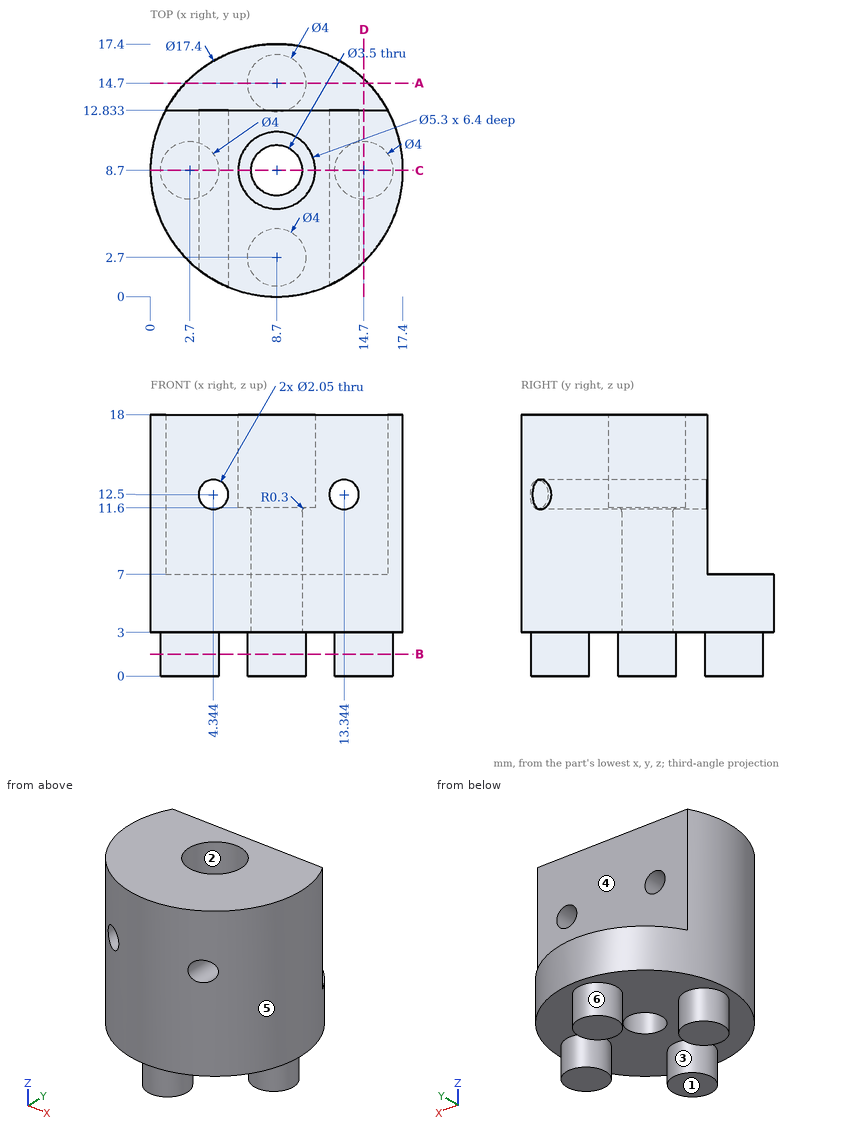
Here's the drawing with two shaded views (mm, measured from the low corner). I have some questions. A direction names the side the tool comes from. Coordinates: 2 decimals unless noted, no trailing zeros. Write each loop counter-clockwise with the first axis right and the second up, starting at its lowest first coordinate (ties: lowest second). Pieces come first, ordered by that corner, then holes. Notation, with made-up numbers: (57.5, 62.25) -> (85.5, 62.25) arc R14 cw to (85.5, 75.25) -> close; hole circle Ø10 at (87, -33.75). An arc over 180 degrees is marked (long way). One line per question, with ' | ' between items. Start each with the question number.
1. If we section it at D-D (x = 14.7): Please give me the cut outline in (y, z).
2. If we section it at C-C (y = 8.7): Count the separate pieces of the cut face and the enclosed holes in it, and give its area (3 significant figures).
3. Thinking about a two-plate mould opening in X: for the marked faces 1, 2 and 3, which applies, pulls with the +X half, pulls with the -X half, needs draft (parallel to the pull), parting line crosses it, or undercut?
4. If we section it at B-B (z = 1.5): Please give me the cut outline in (x, y).
5. For the marked faces 4, 5 and 6, which set-ups out of +Z, -Z, +X, -X, +Y, -Y let a thin tool reach every point of the face, with its end or its side?
6. Will these pins go through, and if not, where does the flat tip stop? P1, Ø2.5, axis at x = 8.5, y = 8.5, coming from the +Z side; P2, Ø1.4, axis at x = 10, y = 14, coming from the +Z side; P3, Ø3, axis at y = 11.5, z = 2, coming from the +X side; P4, Ø4, axis at x = 8.7, y = 8.7, coming from the +Z side.
7. If we section it at A-A (y = 14.7): Please give me the cut outline in (x, z).
8. Please list where these lines run through material, in increasing order: line 1 along Y through (x, z) = (8.7, 7.75); line 2 along X through (y, z) = (6, 12.5); line 3 along Z through (x, y) = (11.5, 8).
Return value:
1) outline: (2.4, 3) -> (6.7, 3) -> (6.7, 0) -> (10.7, 0) -> (10.7, 3) -> (15, 3) -> (15, 7) -> (12.83, 7) -> (12.83, 18) -> (2.4, 18) -> close
2) separate pieces: 2 | enclosed holes: 2 | area: 214 mm²
3) face 1: needs draft | face 2: undercut | face 3: parting line crosses it
4) outline: circle Ø4 at (2.7, 8.7); circle Ø4 at (8.7, 2.7); circle Ø4 at (8.7, 14.7); circle Ø4 at (14.7, 8.7)
5) face 4: +Z, +X, -X, +Y | face 5: +Z, -Z | face 6: -Z
6) P1: passes through | P2: stops at z = 7 | P3: stops at x = 17.24 | P4: stops at z = 11.6
7) outline: (2.4, 3) -> (6.7, 3) -> (6.7, 0) -> (10.7, 0) -> (10.7, 3) -> (15, 3) -> (15, 7) -> (2.4, 7) -> close
8) line 1: y = 0 to 6.95, 10.45 to 12.83 | line 2: x = 0.43 to 3.32, 5.37 to 12.32, 14.37 to 16.97 | line 3: z = 3 to 18
